Read the model definition and answer for the solid it produces. Units are mm, in the model's axes. Coordinates: 2 decimals unless noted, no trailing zeros. Write each loop counter-clockwise with the first axis right and the second up, starting at its lowest first coordinate (ties: lowest second). Pieces come first, ordered by that corner, then holes.
1) The part is cut by section C-C (x = 1). Determine the outline of the cut face in (y, z).
2) The part is cut by section A-A (z = 0). Determine the outline of the cut face in (x, y), then the cut area to 3 significant figures.
3) Each of these flat-tipped pins is pushed along its axis until it touches: pin 1 Ø3 at (x, z) = (-6, 9) entering from -Y; pin 2 Ø12 at (x, z) = (-4.5, 7.5) entering from -Y; pin 3 Ø12 at (x, z) = (-7, 7) entering from +Y. Where does it stop, or does it pass through?
4) Find the intervals of material crossed by line 1 (Y direction, x = 3.75, z = 0); line 2 (Y direction, x = -1, z = -3); line 3 (Z direction, x = -5, y = 7), in increasing order.
5) The part is cut by section D-D (z = 13). Determine the outline of the cut face in (x, y), then the cut area to 3 significant figures.
6) Determine the mould class of faces 1 (the face through (0.14, -15.62, 3.47)), 2 (the face through (-10, 12, -2)), 3 (the face through (-0.14, 0.53, 11.99)) for opening direction Z: +Z half, -Z half, draft (parallel to the pull), parting line (faces both ways), or undercut.
from build123d import *

# Parameters (mm, degrees)
CAGSPISKE_W         = 16
CAGSPISKE_H         = 0.7
SKETCH1_R           = 16
SKETCH1_R_2         = 12
BOSS_EXTRUDE1_DEPTH = 10


with BuildPart() as part:
    # CagSpiSke → CageSpine (revolve)
    with BuildSketch(Plane.XY, mode=Mode.PRIVATE) as cagespine_sk:
        with Locations((0, 14.25)):
            Rectangle(CAGSPISKE_W, CAGSPISKE_H)
    revolve(cagespine_sk.sketch.rotate(Axis((-12.7, 0, 0), (1, 0, 0)), 270), axis=Axis((-12.7, 0, 0), (1, 0, 0)))

    # RolSimSke → RollersSimplified (revolve)
    with BuildSketch(Plane.XY, mode=Mode.PRIVATE) as rollerssimplified_sk:
        with BuildLine():
            Line((-7.13, 16), (7.13, 16))
            ThreePointArc((7.13, 16), (7.179497475, 15.979497475), (7.2, 15.93))
            Line((7.2, 15.93), (7.2, 12.57))
            ThreePointArc((7.2, 12.57), (7.179497475, 12.520502525), (7.13, 12.5))
            Line((7.13, 12.5), (-7.13, 12.5))
            ThreePointArc((-7.13, 12.5), (-7.179497475, 12.520502525), (-7.2, 12.57))
            Line((-7.2, 12.57), (-7.2, 15.93))
            ThreePointArc((-7.2, 15.93), (-7.179497475, 15.979497475), (-7.13, 16))
        make_face()
    revolve(rollerssimplified_sk.sketch.rotate(Axis((-17.78, 0, 0), (1, 0, 0)), 90), axis=Axis((-17.78, 0, 0), (1, 0, 0)))

    # Sketch1 → Boss-Extrude1 (add, symmetric)
    with BuildSketch(Plane(origin=(0, 0, 0), x_dir=(0, 0, -1), z_dir=(1, 0, 0))):
        Circle(SKETCH1_R)
        Circle(SKETCH1_R_2, mode=Mode.SUBTRACT)
    extrude(amount=BOSS_EXTRUDE1_DEPTH, both=True)


solid = part.part
Reported:
1. outline: circle Ø32 at (0, 0); hole circle Ø24 at (0, 0)
2. outline: (-10, -16) - (10, -16) - (10, -12) - (-10, -12) - close; (-10, 12) - (10, 12) - (10, 16) - (-10, 16) - close
2. area: 160 mm2
3. pin 1: stops at y = -14.13
3. pin 2: stops at y = -15.93
3. pin 3: stops at y = 15.97
4. line 1: y = -16 to -12, 12 to 16
4. line 2: y = -15.72 to -11.62, 11.62 to 15.72
4. line 3: z = -14.39 to -9.75, 9.75 to 14.39
5. outline: (-10, -9.33) - (10, -9.33) - (10, 9.33) - (-10, 9.33) - close
5. area: 373 mm2
6. face 1: parting line
6. face 2: draft
6. face 3: undercut
